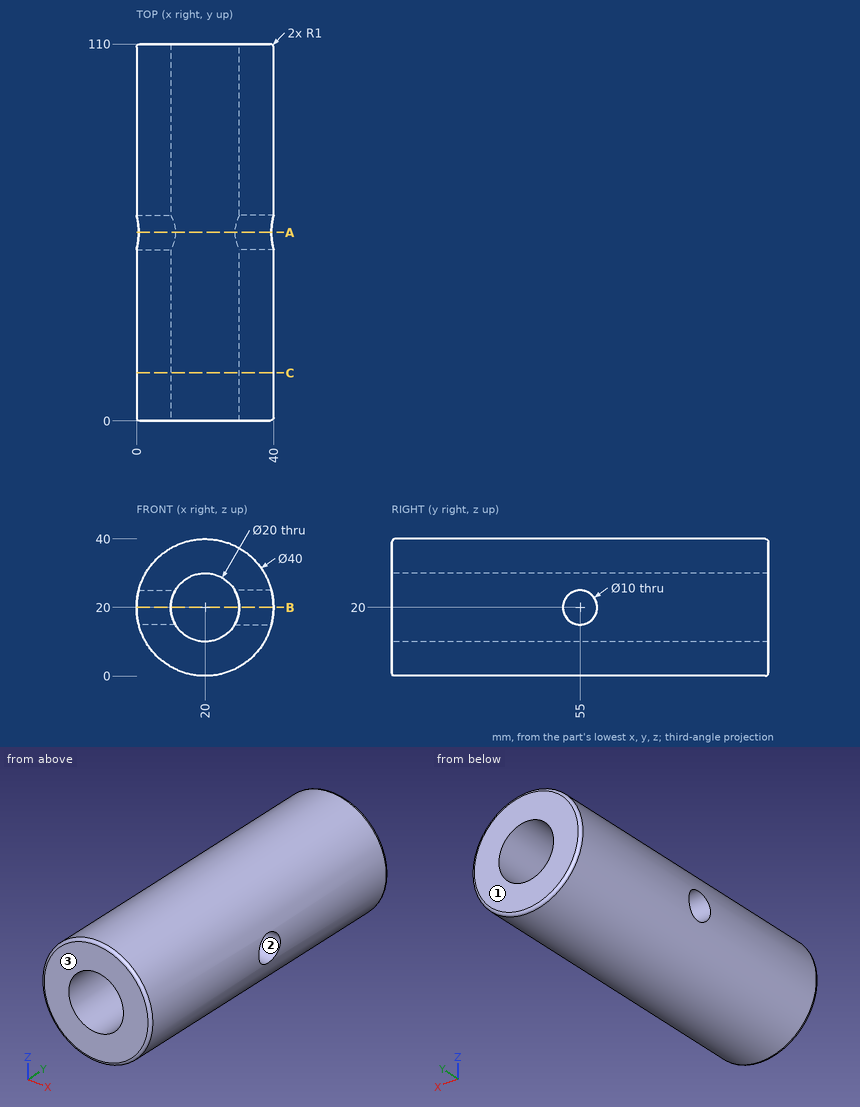
Check sheet for the drawn part. Datum: minimum x, y, z corner. Units: mm. Give positions to 0.01 mm unless a question says otherwise; leave off trailing zeros. Order: outer loops, then holes, each group sorted by start corner. A loop starts at its lowest first (then second) coordinate and runs counter-clockwise, first axis right, second up. Notation, with made-up numbers: (44, 33) -> (51, 33) arc R25 cw to (51, 69) -> close; hole circle Ø9 at (-8.75, 80). An arc over 180 degrees is marked (long way). One line per item, written item: value.
(1) Sectioned sample at A-A on y = 55. Record the cut outline in (x, z).
Final values:
outline: (0.64, 15) arc R20 ccw to (39.36, 15) -> (28.66, 15) arc R10 cw to (11.34, 15) -> close; (0.64, 25) -> (11.34, 25) arc R10 cw to (28.66, 25) -> (39.36, 25) arc R20 ccw to start
(2) Sectioned sample at B-B on z = 20. Count the separate pieces of the cut face and the enclosed holes in it, then the cut area to 3 significant figures.
Final values:
separate pieces: 4
enclosed holes: 0
area: 2,000 mm^2
(3) Gauge pin test, flat ends, axial feed: pin 1 (1 mm diameter, centred on x = 23.5, y = 68.5, fed in from +Z); pin 2 (8 mm diameter, centred on x = 22, y = 18, fed in from +Z); pin 3 (5 mm diameter, centred on x = 16, y = 50.5, fed in from +Z). Record the tip position at first contact, or that the pin passes through.
Final values:
pin 1: z = 39.77
pin 2: z = 40
pin 3: z = 39.94
(4) Draft check along Y on the marked faces 1, 2 and 3. Enter one of: pulls with the +Y half, pulls with the -Y half, needs draft (parallel to the pull), parting line crosses it, or undercut.
Final values:
face 1: pulls with the +Y half
face 2: undercut
face 3: pulls with the -Y half
(5) Scan lines: line 1 along Z through (x, y) = (20, 74); line 2 along X through (y, z) = (82.5, 22); line 3 along Z through (x, y) = (33.5, 52). Record each from-to range of solid material in increasing order. Write a range as [from, to].
Final values:
line 1: [0, 10], [30, 40]
line 2: [0.1, 10.2], [29.8, 39.9]
line 3: [5.24, 16], [24, 34.76]
(6) Sectioned sample at C-C on y = 14. Record the cut outline in (x, z), then the cut area to 3 significant figures.
Final values:
outline: circle Ø40 at (20, 20); hole circle Ø20 at (20, 20)
area: 942 mm^2
